The model under review builds one solid part; all positions refer to its coordinate system, in mm. Coordinates: 2 decimals unless noted, no trailing zeros. Write each loop counter-clockwise with the first axis right and the second up, starting at its lowest first coordinate (ties: lowest second). Pieces come first, ordered by that corner, then holes. Notation, with made-up numbers: (14, 43.5) - (62, 43.5) arc R25 ccw to (62, 55.5) - close; hole circle Ø9 at (-33.5, 19.5). An arc over 180 degrees is marked (long way). Answer as CSV lines item,"result". Start each with the question number.
```python
from build123d import *

# Parameters (mm, degrees)
SZKIC1_W                    = 16
SZKIC1_H                    = 31.855734842
DODANIE_WYCI_GNI_CIE1_DEPTH = 2
SZKIC2_W                    = 16
SZKIC2_H                    = 5
WYTNIJ_WYCI_GNI_CIE1_DEPTH  = 5
WYTNIJ_WYCI_GNI_CIE2_DEPTH  = 10


with BuildPart() as part:
    # Szkic1 → Dodanie-wyciągnięcie1 (new body)
    with BuildSketch(Plane.XY):
        with Locations((8, 15.927867421)):
            Rectangle(SZKIC1_W, SZKIC1_H)
    extrude(amount=DODANIE_WYCI_GNI_CIE1_DEPTH)

    # Szkic2 → Wytnij-wyciągnięcie1 (cut)
    with BuildSketch(Plane.XY.offset(2)):
        with Locations((8, 2.5)):
            Rectangle(SZKIC2_W, SZKIC2_H)
    extrude(amount=-WYTNIJ_WYCI_GNI_CIE1_DEPTH, mode=Mode.SUBTRACT)

    # Szkic6 → Wytnij-wyciągnięcie2 (cut)
    with BuildSketch(Plane(origin=(0, 0, 0), x_dir=(-1, 0, 0), z_dir=(0, 0, -1))):
        with BuildLine():
            Line((0, 31.855734842), (-16, 31.855734842))
            Line((-16, 31.855734842), (-16, 18.750886073))
            ThreePointArc((-16, 18.750886073), (-8.06030582, 15.602264045), (0, 18.427867421))
            Line((0, 18.427867421), (0, 31.855734842))
        make_face()
    extrude(amount=-WYTNIJ_WYCI_GNI_CIE2_DEPTH, mode=Mode.SUBTRACT)


solid = part.part
```
(1) Wall thickness on line 1 (Y direction, x = 7.75, z = 0.2); line 2 (Y direction, x = 10, z = 1.5); line 3 (X direction, y = 16.75, z = 1.6): over which ranges is each line inside the solid? List them lowest first.
(2) Add section A-A on y = 18.25. Give the boundary of the cut face in (x, z).
(3) Add section B-B on z = 0.6. Give the boundary of the cut face in (x, y), then the cut area to 3 significant figures.
(4) Add section C-C on x = 10.75. Give the boundary of the cut face in (y, z).
(5) The part is to be moulded in two halves that separate along X. For faces 1 (the cylindrical face through (8.182, 15.605, 0.986)), 2 (the flat face through (0, 12, 1)), 3 (the flat face through (16, 12, 1)), 4 (the flat face through (8, 10, 0)), say which applies: released by +X, released by -X, zero draft, split by the parting line, or undercut.
Reported:
1,line 1,"5 to 15.6"
1,line 2,"5 to 15.8"
1,line 3,"0 to 2.64, 12.99 to 16"
2,outline,"(0, 0) - (0.22, 0) - (0.22, 2) - (0, 2) - close; (15.41, 0) - (16, 0) - (16, 2) - (15.41, 2) - close"
3,outline,"(0, 5) - (16, 5) - (16, 18.75) arc R12.21 cw to (0, 18.43) - close"
3,area,"185 mm²"
4,outline,"(5, 0) - (15.96, 0) - (15.96, 2) - (5, 2) - close"
5,face 1,"undercut"
5,face 2,"released by -X"
5,face 3,"released by +X"
5,face 4,"zero draft"
